from build123d import *

# Parameters (mm, degrees)
CROQUIS1_R                 = 8
CROQUIS1_R_2               = 3.25
SALIENTE_EXTRUIR1_DEPTH    = 5.5
CORTAR_EXTRUIR1_START      = -3.2
CROQUIS3_R                 = 8.2
CORTAR_EXTRUIR1_DEPTH      = 3.4
CORTAR_EXTRUIR2_DEPTH      = 3.4
CORTAR_EXTRUIR3_REACH      = 16.898
CROQUIS5_R                 = 9
CORTAR_EXTRUIR4_DEPTH      = 13.579745796
CORTAR_EXTRUIR4_DEPTH_BACK = 13.579745796


with BuildPart() as part:
    # Croquis1 → Saliente-Extruir1 (new body)
    with BuildSketch(Plane.XY):
        Circle(CROQUIS1_R)
        Circle(CROQUIS1_R_2, mode=Mode.SUBTRACT)
    extrude(amount=SALIENTE_EXTRUIR1_DEPTH)

    # Croquis3 → Cortar-Extruir1 (cut)
    with BuildSketch(Plane(origin=(0, 6.5, 0), x_dir=(1, 0, 0), z_dir=(0, 1, 0)).offset(CORTAR_EXTRUIR1_START)):
        with Locations((0, 6.632138172)):
            Circle(CROQUIS3_R)
    cortar_extruir1 = extrude(amount=CORTAR_EXTRUIR1_DEPTH, mode=Mode.SUBTRACT)

    # Croquis4 → Cortar-Extruir2 (cut)
    with BuildSketch(Plane(origin=(0, 6.5, 0), x_dir=(1, 0, 0), z_dir=(0, 1, 0))):
        with BuildLine():
            Line((-4.82231721, 1.547107411), (4.82231721, 1.547107411))
            add(Edge.make_bspline(
                [(4.371498599, -0.305440656), (5.098983206, 0.005932333), (5.249256077, 0.623448355), (4.82231721, 1.547107411)],
                knots=[0, 0, 0, 0, 1, 1, 1, 1], degree=3))
            add(Edge.make_bspline(
                [(-4.371498599, -0.305440656), (-2.961142952, -0.90909144), (-0.0365681, -1.156703774), (3.034279152, -0.877788184), (4.371498599, -0.305440656)],
                knots=[0, 0, 0, 0, 0.5, 1, 1, 1, 1], degree=3))
            add(Edge.make_bspline(
                [(-4.371498599, -0.305440656), (-5.098983206, 0.005932333), (-5.249256077, 0.623448355), (-4.82231721, 1.547107411)],
                knots=[0, 0, 0, 0, 1, 1, 1, 1], degree=3))
        make_face()
    cortar_extruir2 = extrude(amount=CORTAR_EXTRUIR2_DEPTH, mode=Mode.SUBTRACT)

    # Simetría1: Cortar-Extruir1, Cortar-Extruir2 across plane
    add(cortar_extruir1.mirror(Plane.ZX), mode=Mode.SUBTRACT)
    add(cortar_extruir2.mirror(Plane.ZX), mode=Mode.SUBTRACT)

    # Cortar-Extruir3: up to this face of the body (flat: up to its plane)
    cortar_extruir3_end = Plane(part.part.faces().sort_by_distance((0, -3.3, 0.632585689))[0])
    # Croquis5 → Cortar-Extruir3 (cut, up to the picked face)
    with BuildSketch(Plane(origin=(0, 3.3, 0), x_dir=(1, 0, 0), z_dir=(0, 1, 0)), mode=Mode.PRIVATE) as cortar_extruir3_sk1:
        with Locations((0, 8.105012001)):
            Circle(CROQUIS5_R)
    cortar_extruir3_tool1 = split(extrude(cortar_extruir3_sk1.sketch, amount=-CORTAR_EXTRUIR3_REACH, mode=Mode.PRIVATE), bisect_by=cortar_extruir3_end, keep=Keep.BOTH, mode=Mode.PRIVATE)
    add(cortar_extruir3_tool1.solids().sort_by(Axis((0, 3.3, -8.105012), (0, -1, 0)))[0], mode=Mode.SUBTRACT)

    # Croquis6 → Cortar-Extruir4 (cut, two sides: drawn at the far end of the back side and taken through both)
    with BuildSketch(Plane(origin=(0, 0, 0), x_dir=(1, 0, 0), z_dir=(0, 1, 0)).offset(-CORTAR_EXTRUIR4_DEPTH_BACK)):
        Polygon((-4.82231721, 0), (-8.482103493, -1.964045705), (-8.482103493, 2.868930537), (8.482103493, 2.868930537), (8.482103493, -1.964045705), (4.82231721, 0), (4.82231721, 1.250339437), (-4.82231721, 1.250339437), align=None)
    extrude(amount=CORTAR_EXTRUIR4_DEPTH + CORTAR_EXTRUIR4_DEPTH_BACK, mode=Mode.SUBTRACT)


solid = part.part
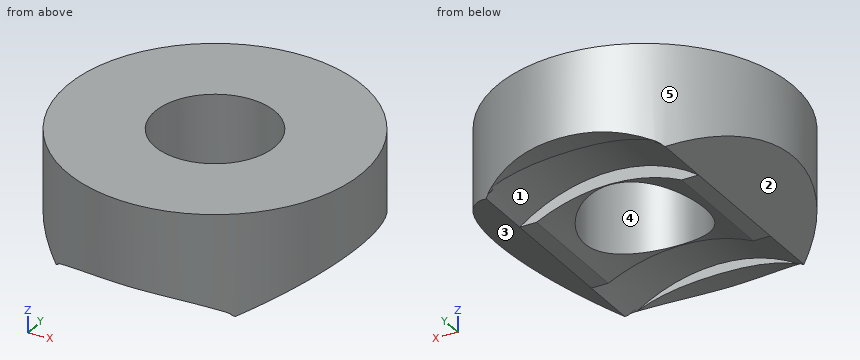
Read the model definition and answer for the solid it produces. Units are mm, in the model's axes. Face numbers are marked on the shaded views. A direction names the side the tool comes from. Coordinates: 2 decimals unless noted, no trailing zeros. Write each loop counter-clockwise with the first axis right and the second up, starting at its lowest first coordinate (ties: lowest second). Pieces come first, ordered by that corner, then holes. Notation, with made-up numbers: (-34.75, 20) -> (-4.75, 20) arc R7 ccw to (-4.75, 24) -> close; hole circle Ø7 at (-35, 61.25). An arc over 180 degrees is marked (long way). Return JSON: item names as keys, results as strings.
(1) For a pull along X with two mould halves and no side action, classify the marked faces 3, 4 and 5 as pulls with the +X half, pulls with the -X half, needs draft (parallel to the pull), parting line crosses it, or undercut.
Answers below:
{"face 3": "pulls with the +X half", "face 4": "undercut", "face 5": "parting line crosses it"}
(2) The part is cut by section D-D on y = 2.75. Give the vertices of the cut face in (x, z), then the cut area to 3 significant figures.
Answers below:
{"outline": "(-7.51, 1.44) -> (-4.82, 0) -> (-3.91, 0) arc R9 cw to (-1.73, 0.73) -> (-1.73, 5.5) -> (-7.51, 5.5) -> close; (1.73, 0.73) arc R9 cw to (3.91, 0) -> (4.82, 0) -> (7.51, 1.44) -> (7.51, 5.5) -> (1.73, 5.5) -> close", "area": "57.9 mm^2"}
(3) The part is cut by section B-B on z = 5.1. Give the vertices of the cut face in (x, y).
Answers below:
{"outline": "circle Ø16 at (0, 0); hole circle Ø6.5 at (0, 0)"}
(4) Which of the six approach directions +Z, -Z, +X, -X, +Y, -Y give full straight-line access (tool end or side, diameter ignored) to the marked faces 1 and 2?
Answers below:
{"face 1": "-Z", "face 2": "-Z, -X, +Y, -Y"}
(5) Consider line 1 along X through (y, z) = (0, 2.3); line 2 along X through (y, z) = (-6.5, 2.85). Determine where each line is inside the solid, lowest interval first. Write a range as from..to.
Answers below:
{"line 1": "-8..-3.25, 3.25..8", "line 2": "-4.66..4.66"}
(6) The part is cut by section A-A on y = 0. Give the vertices of the cut face in (x, z), then the cut area to 3 significant figures.
Answers below:
{"outline": "(-8, 1.71) -> (-4.82, 0) -> (-3.91, 0) arc R9 cw to (-3.25, 0.29) -> (-3.25, 5.5) -> (-8, 5.5) -> close; (3.25, 0.29) arc R9 cw to (3.91, 0) -> (4.82, 0) -> (8, 1.71) -> (8, 5.5) -> (3.25, 5.5) -> close", "area": "46.6 mm^2"}
(7) Each of these flat-tipped pins is pushed along its axis until it touches: P1, Ø1, axis at y = -1, z = 1, coming from the +X side; P2, Ø1, axis at y = 4, z = 2, coming from the +X side; P3, Ø3, axis at x = -4.5, z = 4.5, coming from the +Y side. Where does it stop, or does it pass through?
Answers below:
{"P1": "x = 7.62", "P2": "x = 7.19", "P3": "y = 7.42"}
(8) The part is cut by section C-C on y = -3.75. Give the vertices of the cut face in (x, z), then the cut area to 3 significant figures.
Answers below:
{"outline": "(-7.07, 1.2) -> (-4.82, 0) arc R8.2 cw to (4.82, 0) -> (7.07, 1.2) -> (7.07, 5.5) -> (-7.07, 5.5) -> close", "area": "64.7 mm^2"}
